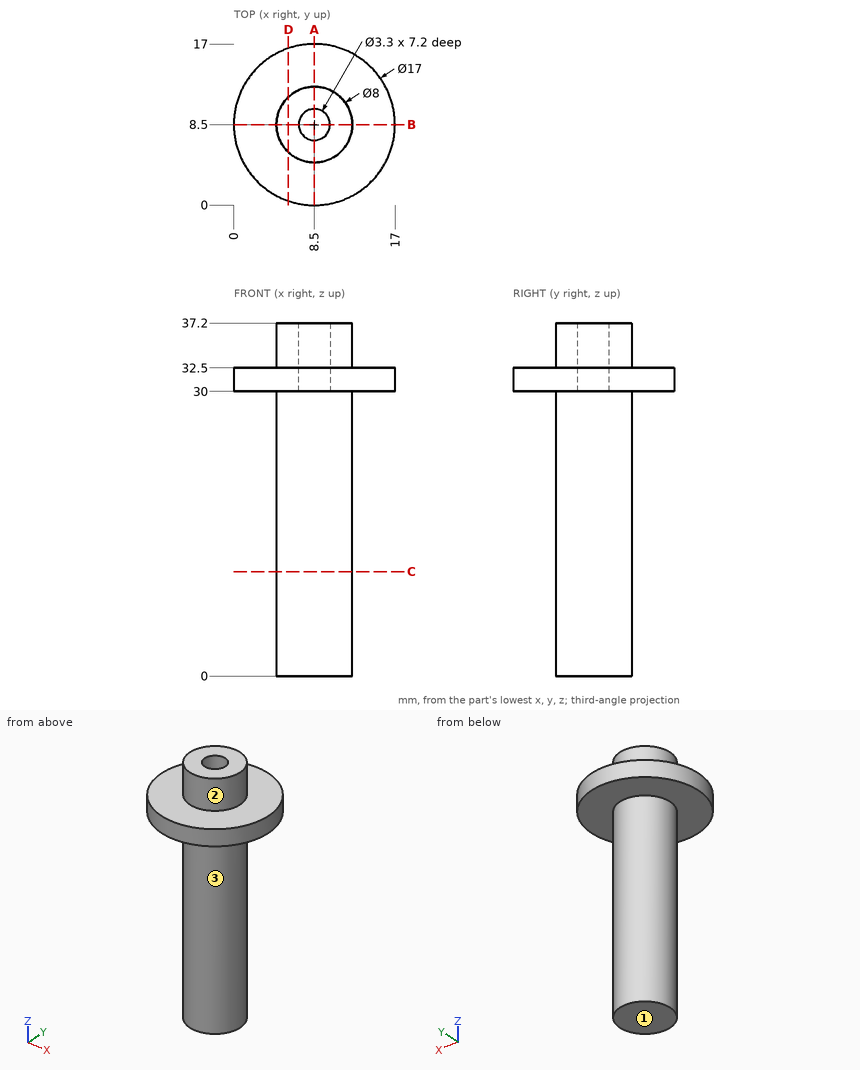
Answer from the drawing. Dimensions are ordinates in mm from the lowest x, y and z of the part. A direction names the side the tool comes from. Coordinates: 2 decimals unless noted, no trailing zeros. Order: outer loops, then holes, each group sorted by start corner. A loop starts at its lowest first (then second) coordinate and runs counter-clockwise, first axis right, second up. Notation, with made-up numbers: (77.25, -30) - (99.25, -30) arc R18 ccw to (99.25, -3) - close; hole circle Ø7 at (-1.75, 51). An arc over 180 degrees is marked (long way). Use one line per item in the form item = value.
(1) Straight lines are drawn through the part: L1, parallel to Y at x = 8.5, z = 35.5; L2, parallel to Z at x = 3.5, y = 13.5; L3, parallel to Y at x = 11, z = 17. For each, find the intervals that lie inside material, in ascending order.
Computed values:
L1 = 4.5 to 6.85, 10.15 to 12.5
L2 = 30 to 32.5
L3 = 5.38 to 11.62
(2) Section A-A, the plane x = 8.5 is taken. Give the vertices of the cut face in (y, z).
Computed values:
outline = (0, 30) - (4.5, 30) - (4.5, 0) - (12.5, 0) - (12.5, 30) - (17, 30) - (17, 32.5) - (12.5, 32.5) - (12.5, 37.2) - (10.15, 37.2) - (10.15, 30) - (6.85, 30) - (6.85, 37.2) - (4.5, 37.2) - (4.5, 32.5) - (0, 32.5) - close
(3) Which of the six approach directions +Z, -Z, +X, -X, +Y, -Y give full straight-line access (tool end or side, diameter ignored) to the marked faces 1, 2 and 3?
Computed values:
face_1 = -Z, +X, -X, +Y, -Y
face_2 = +Z
face_3 = -Z
(4) Section C-C, the plane z = 11 is taken. Give the vertices of the cut face in (x, y), then the cut area to 3 significant figures.
Computed values:
outline = circle Ø8 at (8.5, 8.5)
area = 50.3 mm²
(5) Section D-D, the plane x = 5.75 is taken. Give the vertices of the cut face in (y, z), then the cut area to 3 significant figures.
Computed values:
outline = (0.46, 30) - (5.6, 30) - (5.6, 0) - (11.4, 0) - (11.4, 30) - (16.54, 30) - (16.54, 32.5) - (11.4, 32.5) - (11.4, 37.2) - (5.6, 37.2) - (5.6, 32.5) - (0.46, 32.5) - close
area = 242 mm²
(6) Given pin 1 Ø8 at (x, z) = (15, 22.5) entering from -Y; pin 2 Ø3 at (x, y) = (12, 13) entering from -Z; pin 3 Ø1.5 at (x, y) = (14.5, 2.5) entering from +Z, each flat-ended and moving along its own axis, determine where each tip first touches the part or whether it passes through.
Computed values:
pin_1 = 5.38
pin_2 = 30
pin_3 = 32.5
